Part model, mm, in its own coordinate system. A direction names the side the tool comes from. Coordinates: 2 decimals unless noted, no trailing zeros. Loops run counter-clockwise (first coordinate to the right, second up) from the corner with the lowest first, then second, coordinate; pieces in that order, holes last. Notation, with made-up numbers: M 9.5,72.25 L 34.5,72.25 A22 cw 34.5,100.25 Z; hole C 57.5,45.5 d6. An arc over 180 degrees is marked long. Use a Markdown table: item, result. Add a question column.
1) Pin check, flat tips, straight feed: pin 1 Ø4 at (y, z) = (0, 4) entering from -X; pin 2 Ø12 at (x, y) = (-23.5, -5) entering from +Z; pin 3 Ø6 at (x, y) = (28.57, -10.06) entering from +Z. Stop position of each tip, or through.
2) Band-saw the part on A-A (x = -28.57). List the corners of the cut face in (y, z), plus the area to 3 significant figures.
3) Band-saw the part on D-D (y = 7.5). List the corners of the cut face in (x, z), plus the area to 3 significant figures.
4) Band-saw the part on C-C (x = 4.5). List the corners of the cut face in (y, z).
5) Pull direction X, two halves, no side cores. Call faces 6 (the cylindrical face through (-14.93, 1.72, 9.25)), 7 (the cylindrical face through (-31.068, -9.945, 2.493)), 8 (the flat face through (-38.1, 1.4, 0.5)), 9 (the flat face through (30, -10, 2)): released by +X, released by -X, zero draft, split by the parting line, or undercut.
6) Band-saw the part on B-B (z = 5). List the corners of the cut face in (x, y), plus the area to 3 significant figures.
7) Wall check: probe 1 along Y at (x, z) = (28.57, 1); probe 2 along X at (y, z) = (3, 1.5); probe 3 along Y at (x, z) = (-28.57, 2.45). Give the ranges that are in metal, low to high. Write a range as from..to.
8) Tool access for faces 1 (the flat face through (-1, -8, 3)), 2 (the cylindrical face through (-14.93, -4.07, 3.94)), 3 (the cylindrical face through (-28.92, 1.57, 0.75)), 4 (the cylindrical face through (-14.93, 3.02, 4.43)), 5 (the flat face through (29, 12, 2)): list every direction of +Z, -Z, +X, -X, +Y, -Y with a clear straight run to the whole face (end or side of a thin tool).
from build123d import *

# Parameters (mm, degrees)
F0_W          = 76.2
F0_H          = 30.48
F0_R          = 2.5
F2_DEPTH      = 3
F0_R_2        = 1
F3_DEPTH      = 2
F4_START      = 28.1
F1_R          = 1.5
F4_DEPTH      = 10
F5_START      = -10
F5_DEPTH      = 10
F6_DEPTH      = 10
F6_DEPTH_BACK = 28.1
F7_R          = 1
F8_START      = -20
F8_DEPTH      = 30


with BuildPart() as f2:
    # F0 (on Top) → F2 (new body)
    with BuildSketch(Plane.XY):
        with Locations((0, 1.624652555)):
            Rectangle(F0_W, F0_H)
        with Locations((-28.57, -10.055347445)):
            Circle(F0_R, mode=Mode.SUBTRACT)
        with Locations((28.57, -10.055347445)):
            Circle(F0_R, mode=Mode.SUBTRACT)
        with Locations((-28.57, 13.304652555)):
            Circle(F0_R, mode=Mode.SUBTRACT)
        with Locations((28.57, 13.304652555)):
            Circle(F0_R, mode=Mode.SUBTRACT)
    extrude(amount=F2_DEPTH)

    # F0 (on Top) → F3 (join)
    with BuildSketch(Plane.XY):
        with Locations((28.57, 13.304652555)):
            Circle(F0_R)
        with Locations((28.57, 13.304652555)):
            Circle(F0_R_2, mode=Mode.SUBTRACT)
        with Locations((28.57, -10.055347445)):
            Circle(F0_R)
        with Locations((28.57, -10.055347445)):
            Circle(F0_R_2, mode=Mode.SUBTRACT)
        with Locations((-28.57, -10.055347445)):
            Circle(F0_R)
        with Locations((-28.57, -10.055347445)):
            Circle(F0_R_2, mode=Mode.SUBTRACT)
        with Locations((-28.57, 13.304652555)):
            Circle(F0_R)
        with Locations((-28.57, 13.304652555)):
            Circle(F0_R_2, mode=Mode.SUBTRACT)
    extrude(amount=F3_DEPTH)

    # F1 (on Right) → F4 (join)
    with BuildSketch(Plane.YZ.offset(F4_START)):
        with BuildLine():
            ThreePointArc((-2.5401260508, 5.7960675804), (-4.1005061168, 3.9161569732), (-6.365347445, 3))
            Line((-6.365347445, 3), (-2.115347445, 3))
            ThreePointArc((-2.115347445, 3), (-2.5671360482, 4.3616642469), (-2.5401260508, 5.7960675804))
        make_face()
        with BuildLine():
            Line((5.384652555, 3), (9.634652555, 3))
            ThreePointArc((9.634652555, 3), (7.3698112268, 3.9161569732), (5.8094311608, 5.7960675804))
            ThreePointArc((5.8094311608, 5.7960675804), (5.8658054165, 5.3998067817), (5.884652555, 5))
            ThreePointArc((5.884652555, 5), (5.7577581806, 3.9692235936), (5.384652555, 3))
        make_face()
        with BuildLine():
            ThreePointArc((-2.5401260508, 5.7960675804), (-2.5671360482, 4.3616642469), (-2.115347445, 3))
            Line((-2.115347445, 3), (5.384652555, 3))
            ThreePointArc((5.384652555, 3), (5.7577581806, 3.9692235936), (5.884652555, 5))
            ThreePointArc((5.884652555, 5), (5.8658054165, 5.3998067817), (5.8094311608, 5.7960675804))
            ThreePointArc((5.8094311608, 5.7960675804), (1.634652555, 9.25), (-2.5401260508, 5.7960675804))
        make_face()
        with Locations((1.634652555, 5)):
            Circle(F1_R, mode=Mode.SUBTRACT)
    extrude(amount=F4_DEPTH)

    # F1 (on Right) → F5 (join)
    with BuildSketch(Plane.YZ.offset(F5_START)):
        with BuildLine():
            ThreePointArc((-2.5401260508, 5.7960675804), (-4.1005061168, 3.9161569732), (-6.365347445, 3))
            Line((-6.365347445, 3), (-2.115347445, 3))
            ThreePointArc((-2.115347445, 3), (-2.5671360482, 4.3616642469), (-2.5401260508, 5.7960675804))
        make_face()
        with BuildLine():
            Line((5.384652555, 3), (9.634652555, 3))
            ThreePointArc((9.634652555, 3), (7.3698112268, 3.9161569732), (5.8094311608, 5.7960675804))
            ThreePointArc((5.8094311608, 5.7960675804), (5.8658054165, 5.3998067817), (5.884652555, 5))
            ThreePointArc((5.884652555, 5), (5.7577581806, 3.9692235936), (5.384652555, 3))
        make_face()
        with BuildLine():
            ThreePointArc((-2.5401260508, 5.7960675804), (-2.5671360482, 4.3616642469), (-2.115347445, 3))
            Line((-2.115347445, 3), (5.384652555, 3))
            ThreePointArc((5.384652555, 3), (5.7577581806, 3.9692235936), (5.884652555, 5))
            ThreePointArc((5.884652555, 5), (5.8658054165, 5.3998067817), (5.8094311608, 5.7960675804))
            ThreePointArc((5.8094311608, 5.7960675804), (1.634652555, 9.25), (-2.5401260508, 5.7960675804))
        make_face()
        with Locations((1.634652555, 5)):
            Circle(F1_R, mode=Mode.SUBTRACT)
    extrude(amount=-F5_DEPTH)

    # F1 (on Right) → F6 (cut, two sides)
    with BuildSketch(Plane.YZ) as f6_sk:
        with BuildLine():
            Line((5.384652555, 3), (-2.115347445, 3))
            ThreePointArc((-2.115347445, 3), (1.634652555, 0.75), (5.384652555, 3))
        make_face()
    extrude(amount=-F6_DEPTH, mode=Mode.SUBTRACT)
    extrude(f6_sk.sketch, amount=F6_DEPTH_BACK, mode=Mode.SUBTRACT)

    # F7
    f7_edges = [f2.edges().sort_by_distance(p)[0] for p in [
        (38.1, -13.615347, 1.5),
        (38.1, 16.864653, 1.5),
        (-38.1, 16.864653, 1.5),
        (-38.1, -13.615347, 1.5),
    ]]
    fillet(f7_edges, radius=F7_R)

    # F1 (on Right) → F8 (cut)
    with BuildSketch(Plane.YZ.offset(F8_START)):
        with BuildLine():
            ThreePointArc((-2.5401260508, 5.7960675804), (-2.5671360482, 4.3616642469), (-2.115347445, 3))
            Line((-2.115347445, 3), (5.384652555, 3))
            ThreePointArc((5.384652555, 3), (5.7577581806, 3.9692235936), (5.884652555, 5))
            ThreePointArc((5.884652555, 5), (5.8658054165, 5.3998067817), (5.8094311608, 5.7960675804))
            ThreePointArc((5.8094311608, 5.7960675804), (1.634652555, 9.25), (-2.5401260508, 5.7960675804))
        make_face()
        with Locations((1.634652555, 5)):
            Circle(F1_R, mode=Mode.SUBTRACT)
        with BuildLine():
            Line((5.384652555, 3), (-2.115347445, 3))
            ThreePointArc((-2.115347445, 3), (1.634652555, 0.75), (5.384652555, 3))
        make_face()
    extrude(amount=-F8_DEPTH, mode=Mode.SUBTRACT)


solid = f2.part
Entries:
| question | item | result |
|---|---|---|
| 1 | pin 1 | x = -20 |
| 1 | pin 2 | z = 8.87 |
| 1 | pin 3 | z = 3 |
| 2 | outline | M -13.62,0 L -11.06,0 L -11.06,2 L -12.56,2 L -12.56,3 L -13.62,3 Z; M -9.06,0 L 12.3,0 L 12.3,2 L 10.8,2 L 10.8,3 L 5.38,3 A4.25 cw -2.12,3 L -7.56,3 L -7.56,2 L -9.06,2 Z; M 14.3,0 L 16.86,0 L 16.86,3 L 15.8,3 L 15.8,2 L 14.3,2 Z |
| 2 | area | 61.4 mm2 |
| 3 | outline | M -38.1,0 L 38.1,0 L 38.1,3.82 L 28.1,3.82 L 28.1,3 L -10,3 L -10,3.82 L -20,3.82 L -20,3 L -38.1,3 Z |
| 3 | area | 245 mm2 |
| 4 | outline | M -13.62,0 L 16.86,0 L 16.86,3 L 5.38,3 A4.25 cw -2.12,3 L -13.62,3 Z |
| 5 | face 6 | zero draft |
| 5 | face 7 | undercut |
| 5 | face 8 | released by -X |
| 5 | face 9 | undercut |
| 6 | outline | M -20,-3.02 L -10,-3.02 L -10,0.13 L -20,0.13 Z; M -20,3.13 L -10,3.13 L -10,6.29 L -20,6.29 Z; M 28.1,-3.02 L 38.1,-3.02 L 38.1,0.13 L 28.1,0.13 Z; M 28.1,3.13 L 38.1,3.13 L 38.1,6.29 L 28.1,6.29 Z |
| 6 | area | 126 mm2 |
| 7 | probe 1 | -13.62..-11.06, -9.06..12.3, 14.3..16.86 |
| 7 | probe 2 | -20..-10, 28.1..38.1 |
| 7 | probe 3 | -13.62..-12.56, -7.56..-1.77, 5.03..10.8, 15.8..16.86 |
| 8 | face 1 | +Z, -Y |
| 8 | face 2 | +Z, +X, -X, -Y |
| 8 | face 3 | +Z, -X |
| 8 | face 4 | +X, -X |
| 8 | face 5 | +Z |
